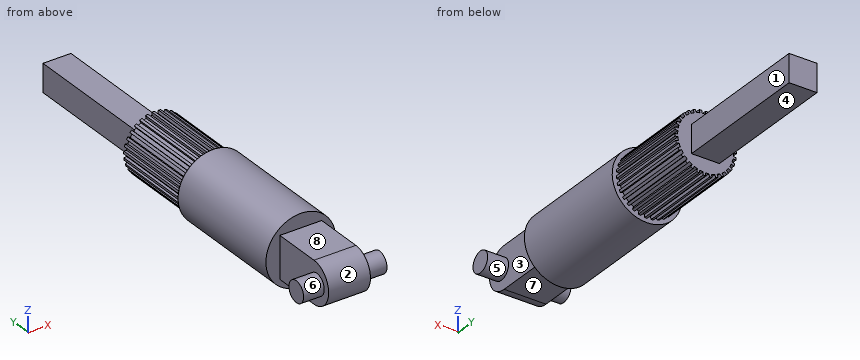
```python
from build123d import *

# Parameters (mm, degrees)
SKETCH1_R                = 2
BOSS_EXTRUDE1_DEPTH      = 6
BOSS_EXTRUDE3_DEPTH      = 6
CIRPATTERN1_COUNT        = 30
SKETCH9_R                = 2.5
BOSS_EXTRUDE5_DEPTH      = 9
SKETCH10_W               = 2
SKETCH10_H               = 2
BOSS_EXTRUDE6_DEPTH      = 10
SKETCH11_W               = 3
SKETCH11_H               = 3
BOSS_EXTRUDE7_DEPTH      = 5
FILLET1_RADIUS           = 1.5
FILLET1_LENGTH           = 3
BOSS_EXTRUDE9_DEPTH      = 1.5
BOSS_EXTRUDE9_DEPTH_BACK = 4.477112072
SKETCH12_R               = 0.75


with BuildPart() as part:
    # Sketch1 → Boss-Extrude1 (new body)
    with BuildSketch(Plane(origin=(0, 0, 0), x_dir=(1, 0, 0), z_dir=(0, 1, 0))):
        with Locations(Location((0, 0, 0), (0, 0, 270))):
            Circle(SKETCH1_R)
    extrude(amount=BOSS_EXTRUDE1_DEPTH)

    # Sketch5 → Boss-Extrude3 (add)
    with BuildSketch(Plane(origin=(0, 6, 0), x_dir=(1, 0, 0), z_dir=(0, 1, 0))):
        Polygon((0, -2), (-0.176506233, -1.992196162), (-0.176506233, -2.202534122), (0, -2.202534122), align=None)
    boss_extrude3 = extrude(amount=-BOSS_EXTRUDE3_DEPTH)

    # CirPattern1: Boss-Extrude3 ×30 about axis
    cirpattern1_axis = Axis((0, 0, 0), (0, 1, 0))
    for i in range(1, CIRPATTERN1_COUNT):
        add(boss_extrude3.rotate(cirpattern1_axis, i * 360 / CIRPATTERN1_COUNT))

    # Sketch9 → Boss-Extrude5 (add)
    with BuildSketch(Plane.XZ):
        with Locations(Location((0, 0, 0), (0, 0, 270))):
            Circle(SKETCH9_R)
    extrude(amount=BOSS_EXTRUDE5_DEPTH)

    # Sketch10 → Boss-Extrude6 (add)
    with BuildSketch(Plane(origin=(0, 6, 0), x_dir=(1, 0, 0), z_dir=(0, 1, 0))):
        with Locations((0.009702593, 0.031661031)):
            Rectangle(SKETCH10_W, SKETCH10_H)
    extrude(amount=BOSS_EXTRUDE6_DEPTH)

    # Sketch11 → Boss-Extrude7 (add)
    with BuildSketch(Plane.XZ.offset(9)):
        Rectangle(SKETCH11_W, SKETCH11_H)
    extrude(amount=BOSS_EXTRUDE7_DEPTH)

    # Fillet1: full round fillet: the end face becomes a half cylinder, R = half its width
    fillet1_face = Plane((0, -14, 0), x_dir=(1, 0, 0), z_dir=(0, -1, 0))  # on the end face: x along it, z out of the body
    fillet1_slab = fillet1_face.offset(-FILLET1_RADIUS / 2) * Box(FILLET1_LENGTH, 2 * FILLET1_RADIUS, FILLET1_RADIUS, mode=Mode.PRIVATE)  # the body's end, R deep
    fillet1_round = Plane((0, -12.5, 0), x_dir=(0, -1, 0), z_dir=(1, 0, 0)) * Cylinder(FILLET1_RADIUS, FILLET1_LENGTH, mode=Mode.PRIVATE)  # its axis R under the face
    add(fillet1_slab - fillet1_round, mode=Mode.SUBTRACT)

    # Sketch12 → Boss-Extrude9 (add, two sides: drawn at the far end of the back side and taken through both)
    with BuildSketch(Plane(origin=(1.5, 0, 0), x_dir=(0, 0, -1), z_dir=(1, 0, 0)).offset(-BOSS_EXTRUDE9_DEPTH_BACK)):
        with Locations((0, -12.8)):
            Circle(SKETCH12_R)
    extrude(amount=BOSS_EXTRUDE9_DEPTH + BOSS_EXTRUDE9_DEPTH_BACK)


solid = part.part
```
Design review of the part built by this model. Coordinates are the model's own, in mm. Face numbers are marked on the shaded views. A direction names the side the tool comes from. Give positions to 0.01 mm unless a question says otherwise; leave off trailing zeros. Order: outer loops, then holes, each group sorted by start corner. A loop starts at its lowest first (then second) coordinate and runs counter-clockwise, first axis right, second up. Notation, with made-up numbers: (32, 47) -> (80, 47) arc R23 ccw to (80, 64) -> close; hole circle Ø2 at (-36, 41). An arc over 180 degrees is marked (long way). Write each question's results on one line, items separated by ' | '. Start each with the question number.
Q1. Wall thickness on L1, parallel to Y at x = 1.8, z = 1.6; L2, parallel to X at y = 9, z = 0.85; L3, parallel to Z at x = 2.6, y = -12.25: over which ranges is each line inside the solid? List them lowest first. Write a range as from..to.
Q2. For pin 1 (1 mm diameter, centred on x = 2, y = 11, fed in from -Z); pin 2 (1.5 mm diameter, centred on y = 8.5, z = -1, fed in from +X); pin 3 (1 mm diameter, centred on x = 0.5, y = 8.5, fed in from -Z); pin 4 (1.5 mm diameter, centred on x = 0, y = -10.5, fed in from +Z), all flat-tipped, find the tip position at first contact; note any pin that passes through.
Q3. Add section C-C on y = -0.25. Give the boundary of the cut face in (x, z), and give its area (3 significant figures).
Q4. Add section A-A on y = 10. Give the boundary of the cut face in (x, z), and give its area (3 significant figures).
Q5. Machinability: for the marked faces 4, 5, 6, 7 and 8, which of the approach directions +Z, -Z, +X, -X, +Y, -Y give a long, thin tool a straight path to every point of the face, cutting with its end or side? Answer none if there is none.
Q6. Add section B-B on y = -12.8. Give the boundary of the cut face in (x, z), and give its area (3 significant figures).
Q7. Mouldability with a two-part tool opening along Y and no side actions: class the marked faces 1, 2 and 3 as +Y half, -Y half, draft (parallel to the pull), parting line (faces both ways), or undercut.
Found:
1) L1: y = -9..0 | L2: x = -0.99..1.01 | L3: z = -0.51..0.51
2) pin 1: passes through | pin 2: stops at x = 1.01 | pin 3: stops at z = -1.03 | pin 4: stops at z = 1.5
3) outline: circle Ø5 at (0, 0) | area: 19.6 mm2
4) outline: (-0.99, -1.03) -> (1.01, -1.03) -> (1.01, 0.97) -> (-0.99, 0.97) -> close | area: 4.00 mm2
5) face 4: -Z, +X, -X, +Y | face 5: +X | face 6: -X | face 7: -Z, +X, -X, -Y | face 8: +Z, +X, -X, -Y
6) outline: (-2.98, -0.75) -> (-1.5, -0.75) -> (-1.5, -1.47) -> (1.5, -1.47) -> (1.5, -0.75) -> (3, -0.75) -> (3, 0.75) -> (1.5, 0.75) -> (1.5, 1.47) -> (-1.5, 1.47) -> (-1.5, 0.75) -> (-2.98, 0.75) -> close | area: 13.3 mm2
7) face 1: draft | face 2: -Y half | face 3: undercut
